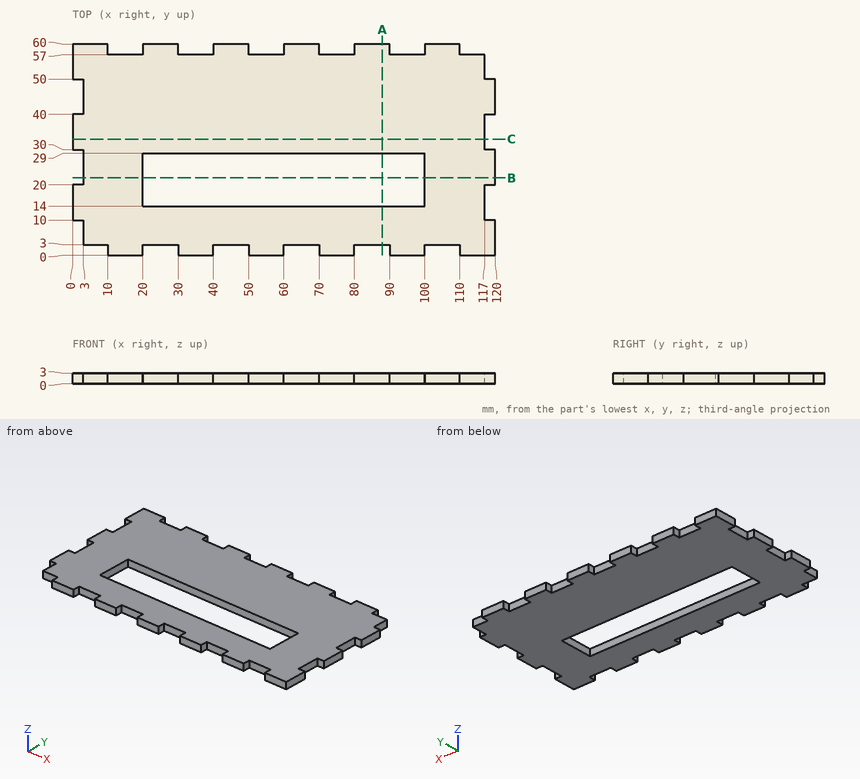
The drawing under review shows one solid part. Ordinate dimensions are in mm from its lowest x, y, z. Coordinates: 2 decimals unless noted, no trailing zeros. Order: outer loops, then holes, each group sorted by start corner. A loop starts at its lowest first (then second) coordinate and runs counter-clockwise, first axis right, second up. Notation, with made-up numbers: (-12.75, -39) - (33.25, -39) arc R33 cw to (33.25, 0) - close; hole circle Ø3 at (-21, 59.25). An arc over 180 degrees is marked (long way). Put each result on its own line as item: value.
1) Insertion check: P1, Ø0.9, axis at x = 118, z = 2, coming from the +Y side; P2, Ø12, axis at x = 28.5, y = 18, coming from the +Z side; P3, Ø1.5, axis at y = 26.5, z = 0.5, coming from the -X side; P4, Ø1.5, axis at y = 58, z = 2, coming from the +X side. Each pin has a flat end and moves straight along its axis. Give the tip position at first contact, or say it passes through.
Response values:
P1: stops at y = 50
P2: stops at z = 3
P3: stops at x = 3
P4: stops at x = 110
2) Wall thickness on L1, parallel to Y at x = 95.5, z = 2.75; L2, parallel to X at y = 16.5, z = 0.8; L3, parallel to Y at x = 84.5, z = 0.55: over which ranges is each line inside the solid? List them lowest first. Write a range as from..to.
Response values:
L1: y = 0..14, 29..57
L2: x = 0..20, 100..117
L3: y = 3..14, 29..60
3) Take a section at A-A, the plane x = 88. Give the boundary of the cut face in (y, z), and give its area (3 significant figures).
Response values:
outline: (3, 0) - (14, 0) - (14, 3) - (3, 3) - close; (29, 0) - (60, 0) - (60, 3) - (29, 3) - close
area: 126 mm²
4) Take a section at B-B, the plane y = 22. Give the boundary of the cut face in (x, z).
Response values:
outline: (3, 0) - (20, 0) - (20, 3) - (3, 3) - close; (100, 0) - (120, 0) - (120, 3) - (100, 3) - close
5) Take a section at C-C, the plane y = 33. Give the boundary of the cut face in (x, z), and give its area (3 significant figures).
Response values:
outline: (0, 0) - (117, 0) - (117, 3) - (0, 3) - close
area: 351 mm²
